from build123d import *

# Parameters (mm, degrees)
SKETCH1_R           = 2.2479
SKETCH1_R_2         = 1.63195
BOSS_EXTRUDE1_DEPTH = 6.477


with BuildPart() as part:
    # Sketch1 → Boss-Extrude1 (new body)
    with BuildSketch(Plane.XY):
        Polygon((-6.985, -107.823), (-1.27, -107.823), (-1.27, -101.473), (-3.175, -101.473), (-3.175, -98.933), (-1.27, -98.933), (-1.27, -95.123), (1.27, -95.123), (1.27, -98.933), (3.175, -98.933), (3.175, -101.473), (1.27, -101.473), (1.27, -107.823), (6.985, -107.823), (6.985, -114.3), (40.894, -114.3), (40.894, 114.3), (6.985, 114.3), (6.985, 107.823), (1.27, 107.823), (1.27, 101.473), (3.175, 101.473), (3.175, 98.933), (1.27, 98.933), (1.27, 95.123), (-1.27, 95.123), (-1.27, 98.933), (-3.175, 98.933), (-3.175, 101.473), (-1.27, 101.473), (-1.27, 107.823), (-6.985, 107.823), (-6.985, 114.3), (-40.894, 114.3), (-40.894, -114.3), (-6.985, -114.3), align=None)
        with Locations((-25.654, -101.6)):
            Circle(SKETCH1_R, mode=Mode.SUBTRACT)
        with Locations((-20.447, -111.0615)):
            Circle(SKETCH1_R_2, mode=Mode.SUBTRACT)
        with Locations((20.447, -111.0615)):
            Circle(SKETCH1_R_2, mode=Mode.SUBTRACT)
        with Locations((25.654, -101.6)):
            Circle(SKETCH1_R, mode=Mode.SUBTRACT)
        with Locations((-25.654, 101.6)):
            Circle(SKETCH1_R, mode=Mode.SUBTRACT)
        with Locations((-20.447, 111.0615)):
            Circle(SKETCH1_R_2, mode=Mode.SUBTRACT)
        with Locations((20.447, 111.0615)):
            Circle(SKETCH1_R_2, mode=Mode.SUBTRACT)
        with Locations((25.654, 101.6)):
            Circle(SKETCH1_R, mode=Mode.SUBTRACT)
    extrude(amount=BOSS_EXTRUDE1_DEPTH)


solid = part.part
Geometry: final body of the model. Coordinates: model frame, mm. A direction names the side the tool comes from. Round coordinates to 2 decimals unless told otherwise and drop trailing zeros.
Q1. Access query for faces 1 (the flat face through (-1.27, 97, 3)), 2 (the flat face through (-1, 2, 0)), 3 (the flat face through (-1.27, -105, 3)). Directions: +Z, -Z, +X, -X, +Y, -Y. A direction counts if a zero-diameter tool reaches every point of the face in a straight line with its end or side. Return the directions, or none.
Q2. Section A-A on z = 2.75. State how many separate pieces and enclosed holes the cut face has, plus the area to 3 significant figures.
Q3. Material intervals for L1, parallel to Y at x = -3, z = 2; L2, parallel to Y at x = 19, z = 2.75; L3, parallel to Y at x = -6, z = 3.75, sorted ascending.
Q4. Pin query (flat end, axial travel): P1, Ø1, axis at x = -2, z = 3.5, coming from the +Y side; P2, Ø3.5, axis at x = -25.654, y = 101.6, coming from the -Z side; P3, Ø0.6, axis at x = -2, z = 4.5, coming from the -Y side; P4, Ø1.3, axis at x = 0.5, z = 2, coming from the -Y side. Return the tip coordinate at first contact, or that it passes through.
Q5. Pull-direction query (X, two-part tool) for faces 4 (the cylindrical face through (23.87, 100.23, 3.19)), 5 (the flat face through (-1.27, 105, 3)), 6 (the flat face through (24, 114.3, 3)), 7 (the flat face through (-40.894, 2, 3)); classes: released by +X, released by -X, zero draft, split by the parting line, or undercut.
Evaluation:
1. face 1: +Z, -Z, +Y
1. face 2: -Z, +X, -X, +Y, -Y
1. face 3: +Z, -Z, -Y
2. separate pieces: 1
2. enclosed holes: 8
2. area: 18,300 mm2
3. L1: y = -107.82 to -101.47, -98.93 to 98.93, 101.47 to 107.82
3. L2: y = -114.3 to -111.82, -110.31 to 110.31, 111.82 to 114.3
3. L3: y = -107.82 to 107.82
4. P1: stops at y = 107.82
4. P2: passes through
4. P3: stops at y = -107.82
4. P4: stops at y = -95.12
5. face 4: undercut
5. face 5: undercut
5. face 6: zero draft
5. face 7: released by -X
